Work out the finished part from the listing and answer in its coordinate system (mm). A direction names the side the tool comes from. Give positions to 0.01 mm unless a question says otherwise; leave off trailing zeros. Order: outer loops, then holes, each group sorted by start corner. A loop starts at its lowest first (then second) coordinate and runs counter-clockwise, first axis right, second up. Notation, with made-up numbers: (16.25, 14.5) - (54.25, 14.5) arc R16 ccw to (54.25, 20.5) - close; hole circle Ø8 at (-5, -8.5). An arc over 180 degrees is marked (long way). Put each result on its own line as item: value.
```python
from build123d import *

# Parameters (mm, degrees)
EXTRUDE1_DEPTH = 3.81


with BuildPart() as part:
    # Sketch1 → Revolve1 (revolve)
    with BuildSketch(Plane.XY, mode=Mode.PRIVATE) as revolve1_sk:
        Polygon((25.3365, 0), (25.3365, 2.31775), (24.54275, 3.1115), (-19.1135, 3.1115), (-19.1135, 4.191), (-19.6215, 4.699), (-24.8285, 4.699), (-25.3365, 4.191), (-25.3365, 0), align=None)
    revolve(revolve1_sk.sketch.rotate(Axis((-124.874669814, 0, 0), (1, 0, 0)), 90), axis=Axis((-124.874669814, 0, 0), (1, 0, 0)))

    # Sketch2 → Extrude1 (cut)
    with BuildSketch(Plane.ZY.offset(25.3365)):
        Polygon((0, 2.749630657), (-2.38125, 1.374815329), (-2.38125, -1.374815329), (0, -2.749630657), (2.38125, -1.374815329), (2.38125, 1.374815329), align=None)
    extrude(amount=-EXTRUDE1_DEPTH, mode=Mode.SUBTRACT)


solid = part.part
```
(1) Section C-C, the plane x = 15.5 is taken. Write down the section's boundary in (y, z).
Geometry check:
outline: circle Ø6.22 at (0, 0)
(2) Section B-B, the plane y = 0 is taken. Write down the section's boundary in (x, z).
Geometry check:
outline: (-25.34, -4.19) - (-24.83, -4.7) - (-19.62, -4.7) - (-19.11, -4.19) - (-19.11, -3.11) - (24.54, -3.11) - (25.34, -2.32) - (25.34, 2.32) - (24.54, 3.11) - (-19.11, 3.11) - (-19.11, 4.19) - (-19.62, 4.7) - (-24.83, 4.7) - (-25.34, 4.19) - (-25.34, 2.38) - (-21.53, 2.38) - (-21.53, -2.38) - (-25.34, -2.38) - close
(3) Straight lines are drawn through the part: line 1 (X direction, y = 1.75, z = -3.75); line 2 (Y direction, x = 12.5, z = 0); line 3 (Y direction, x = 20, z = -2). For each, find the intervals that lie inside material, in ascending order.
Geometry check:
line 1: x = -25.34 to -19.11
line 2: y = -3.11 to 3.11
line 3: y = -2.38 to 2.38
(4) A tool of negligible diameter and unlimited length cuts with its end or side. For faces 4 (the face through (-25.336, 2, 2)), 5 (the face through (2.41, 2.76, 1.44)), 6 (the face through (-23.458, 2.072, -1.174)), from which of +Z, -Z, +X, -X, +Y, -Y can it reach the whole face along a straight path? Write none if from no direction.
Geometry check:
face 4: +Z, -Z, -X, +Y, -Y
face 5: +X
face 6: -X
(5) Given pin 1 (3 mm diameter, centred on x = -2, y = 1, fed in from +Z); pin 2 (3 mm diameter, centred on x = -24, y = -0.5, fed in from +Z); pin 3 (2 mm diameter, centred on x = 3, y = -2.5, fed in from +Z); pin 4 (1 mm diameter, centred on x = -6, z = 0.5, fed in from -Y), each flat-ended and moving along its own axis, determine where each tip first touches the part or whether it passes through.
Geometry check:
pin 1: stops at z = 3.11
pin 2: stops at z = 4.7
pin 3: stops at z = 2.73
pin 4: stops at y = -3.11
(6) Section A-A, the plane x = -22 is taken. Write down the section's boundary in (y, z), then the cut area to 3 significant figures.
Geometry check:
outline: circle Ø9.4 at (0, 0); hole (-2.75, 0) - (-1.37, -2.38) - (1.37, -2.38) - (2.75, 0) - (1.37, 2.38) - (-1.37, 2.38) - close
area: 49.7 mm²
(7) Determine the mould class of faces 1 (the face through (-19.114, 2, 3)), 2 (the face through (-23, 0, 2.381)), 3 (the face through (-22.26, -4.66, -0.61)) for opening direction Z: pulls with the +Z half, pulls with the -Z half, needs draft (parallel to the pull), parting line crosses it, or undercut.
Geometry check:
face 1: needs draft
face 2: undercut
face 3: parting line crosses it
